The model under review builds one solid part; all positions refer to its coordinate system, in mm. A direction names the side the tool comes from. Round coordinates to 2 decimals unless told otherwise and drop trailing zeros. Loops run counter-clockwise (first coordinate to the right, second up) from the corner with the lowest first, then second, coordinate; pieces in that order, holes last. Notation, with made-up numbers: M 17.25,5.5 L 40.25,5.5 A28 cw 40.25,28.5 Z; hole C 70,-8 d5. An arc over 180 degrees is marked long. Return JSON: item names as keys, results as strings. Group by question number.
Q1. Consider section A-A (z = 0). State the section outline as (x, y) points, and give its area (3 significant figures).
Q2. For faces 1 (the face through (-1.71, 16.97, -0.38)), 2 (the face through (1.17, 7.4, -1.98)), list the 3-axis set-ups (+Z, -Z, +X, -X, +Y, -Y) from which the entire face can be reached by the end or side of a thin tool; tool diameter is ignored.
Q3. Consider section D-D (z = 2). State the section outline as (x, y) points.
Q4. Consider section C-C (x = -0.5). State the section outline as (y, z) points, and give its area (3 significant figures).
Q5. Consider section B-B (y = 4.5). State the section outline as (x, z) points, and give its area (3 significant figures).
Q6. Draft analysis for pull direction Z (two halves, no side actions). For faces 3 (the face through (-1.17, 7.4, 1.98)), 4 (the face through (2.3, 7, 0)), 5 (the face through (0.27, 9.37, 1.22)), state which applies: pulls with the +Z half, pulls with the -Z half, needs draft (parallel to the pull), parting line crosses it, or undercut.
Q7. Clearance check with a flat-ended pin moving along its axis: pin 1 Ø1.5 at (x, y) = (-1.5, 4) entering from +Z. State where the tip first meets the part, or that it passes through.
Q8. To check wall thickness, follow line 1 along X through (y, z) = (13.25, -0.1); line 2 along Y through (x, z) = (-1.65, 1.2); line 3 along Z through (x, y) = (-1, 16). State the ranges of each line that lie inside material, in increasing order.
from build123d import *

# Parameters (mm, degrees)
EXTRUDE_1_DEPTH    = 15
SKETCH_2_R         = 1.75
EXTRUDE_2_DEPTH    = 4
HOLE_WIZARD_M3_1_D = 2.5


with BuildPart() as part:
    # 草图1 → 凸台-拉伸1 (new body)
    with BuildSketch(Plane(origin=(0, 0, 0), x_dir=(1, 0, 0), z_dir=(0, 1, 0))):
        Polygon((0, 2.655811238), (-2.3, 1.327905619), (-2.3, -1.327905619), (0, -2.655811238), (2.3, -1.327905619), (2.3, 1.327905619), align=None)
    extrude(amount=EXTRUDE_1_DEPTH)

    # 草图2 → 凸台-拉伸2 (add)
    with BuildSketch(Plane(origin=(0, 15, 0), x_dir=(1, 0, 0), z_dir=(0, 1, 0))):
        with Locations(Location((0, 0, 0), (0, 0, 270))):
            Circle(SKETCH_2_R)
    extrude(amount=EXTRUDE_2_DEPTH)

    # M3 螺纹孔1 (through all)
    with Locations(Plane(origin=(0, 19, 0), x_dir=(1, 0, 0), z_dir=(0, 1, 0))):
        with Locations((0, 0)):
            Hole(HOLE_WIZARD_M3_1_D / 2)


solid = part.part
Values:
{
 "1": {"outline": "M -2.3,0 L -1.25,0 L -1.25,19 L -1.75,19 L -1.75,15 L -2.3,15 Z; M 1.25,0 L 2.3,0 L 2.3,15 L 1.75,15 L 1.75,19 L 1.25,19 Z", "area": "35.5 mm2"},
 "2": {"face 1": "+Y", "face 2": "-Z, +X, +Y, -Y"},
 "3": {"outline": "M -1.14,0 L 1.14,0 L 1.14,15 L -1.14,15 Z"},
 "4": {"outline": "M 0,-2.37 L 15,-2.37 L 15,-1.68 L 19,-1.68 L 19,-1.15 L 0,-1.15 Z; M 0,1.15 L 19,1.15 L 19,1.68 L 15,1.68 L 15,2.37 L 0,2.37 Z", "area": "40.9 mm2"},
 "5": {"outline": "M -2.3,-1.33 L 0,-2.66 L 2.3,-1.33 L 2.3,1.33 L 0,2.66 L -2.3,1.33 Z; hole C 0,0 d2.5", "area": "13.4 mm2"},
 "6": {"face 3": "pulls with the +Z half", "face 4": "needs draft", "face 5": "undercut"},
 "7": {"pin 1": "stops at z = 2.22"},
 "8": {"line 1": "x = -2.3 to -1.25, 1.25 to 2.3", "line 2": "y = 0 to 15", "line 3": "z = -1.44 to -0.75, 0.75 to 1.44"}
}
